Model file for the job. Use its own axes, mm. Coordinates: 2 decimals unless noted, no trailing zeros. Order: outer loops, then holes, each group sorted by start corner. A loop starts at its lowest first (then second) coordinate and runs counter-clockwise, first axis right, second up. Notation, with made-up numbers: (-7, 21.5) -> (48, 21.5) arc R9 cw to (48, 26.5) -> close; hole circle Ø6 at (85.5, 57.5). An arc over 180 degrees is marked (long way). Return JSON: item names as keys, results as strings. Group by question number.
1) Cut at B-B (z = 7). Write the cut outline in (x, y).
2) Cut at C-C (x = -23). Write the cut outline in (y, z), and give its area (3 significant figures).
3) Probe line 1 (Z direction, x = -20, y = -7.5); line 2 (X direction, y = -18.25, z = -1.5); line 3 (Z direction, x = 0, y = -8.75) (3 decimals). List the from-to ranges inside material, lowest first.
4) Flat gauge pins, fed straight in: pin 1 (8 mm diameter, centred on x = -3.5, y = -9, fed in from +Z); pin 2 (6 mm diameter, centred on x = -4.5, y = -14.5, fed in from -Z); pin 3 (5 mm diameter, centred on y = -5, z = -3, fed in from -X); pin 4 (5 mm diameter, centred on x = 0, z = 0, fed in from +Y). Where does each tip first touch, or does it go through?
5) Cut at A-A (x = -2.5). Write the cut outline in (y, z).
from build123d import *

# Parameters (mm, degrees)
SKETCH1_W               = 123.825
SKETCH1_H               = 25.4
SKETCH2_OUTSIDE_W       = 328.022
SKETCH2_OUTSIDE_H       = 328.022
CUT_EXTRUDE1_DEPTH      = 10
CUT_EXTRUDE1_DEPTH_BACK = 35.4


with BuildPart() as part:
    # Sketch1 → Revolve1 (revolve)
    with BuildSketch(Plane.XY):
        with Locations((65.0875, -12.7)):
            Rectangle(SKETCH1_W, SKETCH1_H)
    revolve(axis=Axis((0, -1254, 0), (0, 1, 0)))

    # Sketch2 outside → Cut-Extrude1 (cut, two sides)
    with BuildSketch(Plane(origin=(0, 0, 0), x_dir=(1, 0, 0), z_dir=(0, 1, 0))) as cut_extrude1_sk:
        Rectangle(SKETCH2_OUTSIDE_W, SKETCH2_OUTSIDE_H)
        with BuildLine():
            ThreePointArc((6.35, 0), (6.329912836, 1.284135818), (6.27254171, 2.56714667))
            ThreePointArc((6.27254171, 2.56714667), (6.175326887, 3.824361251), (6.03246285, 5.077209643))
            ThreePointArc((6.03246285, 5.077209643), (5.842143008, 6.297144559), (5.595092591, 7.506867226))
            ThreePointArc((5.595092591, 7.506867226), (5.286100034, 8.696690934), (4.908320284, 9.866494044))
            ThreePointArc((4.908320284, 9.866494044), (4.445694933, 11.036480903), (3.903262447, 12.17167184))
            ThreePointArc((3.903262447, 12.17167184), (3.246006434, 13.319190062), (2.500680026, 14.411559999))
            ThreePointArc((2.500680026, 14.411559999), (1.608536581, 15.51119354), (0.624958662, 16.529863421))
            ThreePointArc((0.624958662, 16.529863421), (-0.532205476, 17.53111816), (-1.776823287, 18.421323977))
            ThreePointArc((-1.776823287, 18.421323977), (-3.209328759, 19.252740722), (-4.715795066, 19.941133777))
            ThreePointArc((-4.715795066, 19.941133777), (-6.406453621, 20.519055391), (-8.146794068, 20.923449837))
            ThreePointArc((-8.146794068, 20.923449837), (-10.046848772, 21.163603755), (-11.961570845, 21.205090642))
            ThreePointArc((-11.961570845, 21.205090642), (-13.991121641, 21.035122659), (-15.99114089, 20.650559852))
            ThreePointArc((-15.99114089, 20.650559852), (-18.044142393, 20.021705604), (-20.01719815, 19.174755893))
            ThreePointArc((-20.01719815, 19.174755893), (-21.970442626, 18.071028594), (-23.791190022, 16.760205626))
            ThreePointArc((-23.791190022, 16.760205626), (-25.516143096, 15.203834234), (-27.05861892, 13.466444423))
            ThreePointArc((-27.05861892, 13.466444423), (-28.434599881, 11.518792927), (-29.585456445, 9.430205097))
            ThreePointArc((-29.585456445, 9.430205097), (-30.512481977, 7.187988004), (-31.183290683, 4.85626557))
            ThreePointArc((-31.183290683, 4.85626557), (-31.593025755, 2.44288094), (-31.75, 0))
            ThreePointArc((-31.75, 0), (-31.593025755, -2.44288094), (-31.183290683, -4.85626557))
            ThreePointArc((-31.183290683, -4.85626557), (-30.512481977, -7.187988004), (-29.585456445, -9.430205097))
            ThreePointArc((-29.585456445, -9.430205097), (-28.434599881, -11.518792927), (-27.05861892, -13.466444423))
            ThreePointArc((-27.05861892, -13.466444423), (-25.516143096, -15.203834234), (-23.791190022, -16.760205626))
            ThreePointArc((-23.791190022, -16.760205626), (-21.970442626, -18.071028594), (-20.01719815, -19.174755893))
            ThreePointArc((-20.01719815, -19.174755893), (-18.044142393, -20.021705604), (-15.99114089, -20.650559852))
            ThreePointArc((-15.99114089, -20.650559852), (-13.991121641, -21.035122659), (-11.961570845, -21.205090642))
            ThreePointArc((-11.961570845, -21.205090642), (-10.046848772, -21.163603755), (-8.146794068, -20.923449837))
            ThreePointArc((-8.146794068, -20.923449837), (-6.406453621, -20.519055391), (-4.715795066, -19.941133777))
            ThreePointArc((-4.715795066, -19.941133777), (-3.209328759, -19.252740722), (-1.776823287, -18.421323977))
            ThreePointArc((-1.776823287, -18.421323977), (-0.532205476, -17.53111816), (0.624958662, -16.529863421))
            ThreePointArc((0.624958662, -16.529863421), (1.608536581, -15.51119354), (2.500680026, -14.411559999))
            ThreePointArc((2.500680026, -14.411559999), (3.246006434, -13.319190062), (3.903262447, -12.17167184))
            ThreePointArc((3.903262447, -12.17167184), (4.445694933, -11.036480903), (4.908320284, -9.866494044))
            ThreePointArc((4.908320284, -9.866494044), (5.286100034, -8.696690934), (5.595092591, -7.506867226))
            ThreePointArc((5.595092591, -7.506867226), (5.842143008, -6.297144559), (6.03246285, -5.077209643))
            ThreePointArc((6.03246285, -5.077209643), (6.175326887, -3.824361251), (6.27254171, -2.56714667))
            ThreePointArc((6.27254171, -2.56714667), (6.329912836, -1.284135818), (6.35, 0))
        make_face(mode=Mode.SUBTRACT)
    extrude(amount=CUT_EXTRUDE1_DEPTH, mode=Mode.SUBTRACT)
    extrude(cut_extrude1_sk.sketch, amount=-CUT_EXTRUDE1_DEPTH_BACK, mode=Mode.SUBTRACT)


solid = part.part
Answers below:
{
 "1": {"outline": "(-30.58, -25.4) -> (5.71, -25.4) -> (5.71, 0) -> (-30.58, 0) -> close"},
 "2": {"outline": "(-25.4, -17.37) -> (0, -17.37) -> (0, 17.37) -> (-25.4, 17.37) -> close", "area": "882 mm^2"},
 "3": {"line 1": "z = -19.18 to 19.18", "line 2": "x = -31.68 to -2.8, 2.8 to 6.32", "line 3": "z = -17.094 to -3.175, 3.175 to 17.094"},
 "4": {"pin 1": "stops at z = 20.79", "pin 2": "stops at z = -20.79", "pin 3": "stops at x = -31.74", "pin 4": "passes through"},
 "5": {"outline": "(-25.4, -18.86) -> (0, -18.86) -> (0, -1.96) -> (-25.4, -1.96) -> close; (-25.4, 1.96) -> (0, 1.96) -> (0, 18.86) -> (-25.4, 18.86) -> close"}
}
